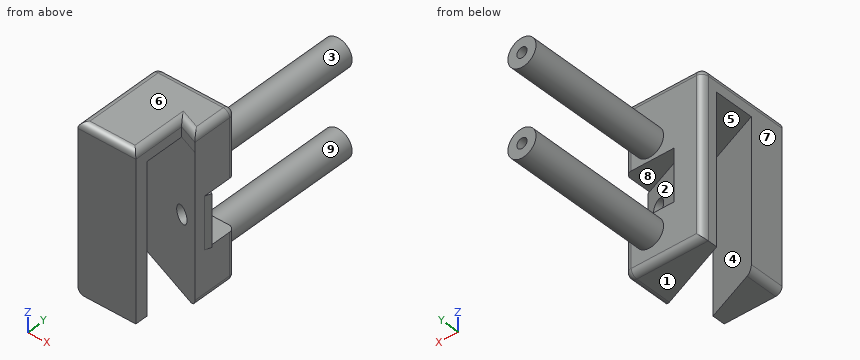
```python
from build123d import *

# Parameters (mm, degrees)
BOSS_EXTRUDE1_DEPTH  = 58.42
SKETCH2_W            = 22.86
SKETCH2_H            = 29.69248518
BOSS_EXTRUDE2_DEPTH  = 6.35
BOSS_EXTRUDE3_DEPTH  = 58.42
CUT_EXTRUDE1_DEPTH   = 58.42
BOSS_EXTRUDE5_DEPTH  = 19.05
BOSS_EXTRUDE6_DEPTH  = 19.05
SKETCH8_R            = 3.3
CUT_EXTRUDE2_DEPTH   = 4.085289
SKETCH9_R            = 5.55625
BOSS_EXTRUDE7_DEPTH  = 64.262
SKETCH11_R           = 1.999996
CUT_EXTRUDE3_DEPTH   = 6.99999997
BOSS_EXTRUDE8_DEPTH  = 6.35
BOSS_EXTRUDE9_DEPTH  = 6.35
FILLET3_R            = 2.54
BOSS_EXTRUDE10_START = 2.54
SKETCH15_W           = 20.926247949
SKETCH15_H           = 20.32
SKETCH15_R           = 3.3
BOSS_EXTRUDE10_DEPTH = 2.54


with BuildPart() as part:
    # Sketch1 → Boss-Extrude1 (new body)
    with BuildSketch(Plane.XY):
        Polygon((0, 0), (22.86, 0), (22.86, 5.08), (0, 13.97), align=None)
    extrude(amount=BOSS_EXTRUDE1_DEPTH)

    # Sketch2 → Boss-Extrude2 (add)
    with BuildSketch(Plane.XY.offset(58.42)):
        with Locations((11.43, 14.84624259)):
            Rectangle(SKETCH2_W, SKETCH2_H)
    extrude(amount=BOSS_EXTRUDE2_DEPTH)

    # Sketch3 → Boss-Extrude3 (add)
    with BuildSketch(Plane(origin=(0, 0, 58.42), x_dir=(-1, 0, 0), z_dir=(0, 0, -1))):
        Polygon((-22.86, 29.69248518), (0, 29.69248518), (-30.774794254, 17.724509637), (-30.774794254, 29.69248518), align=None)
    extrude(amount=BOSS_EXTRUDE3_DEPTH)

    # Sketch5 → Cut-Extrude1 (cut)
    with BuildSketch(Plane(origin=(0, 0, 0), x_dir=(-1, 0, 0), z_dir=(0, 0, -1))):
        Polygon((-30.774794254, 22.107844851), (-11.271433408, 29.69248518), (-30.774794254, 29.69248518), align=None)
    extrude(amount=-CUT_EXTRUDE1_DEPTH, mode=Mode.SUBTRACT)

    # Sketch7 → Boss-Extrude6 (add)
    with BuildSketch(Plane.XY.offset(58.42)):
        Polygon((30.774794254, 22.107844851), (30.774794254, 29.69248518), (11.271433408, 29.69248518), align=None)
    extrude(amount=-BOSS_EXTRUDE6_DEPTH)

    # Sketch8 → Cut-Extrude2 (cut)
    with BuildSketch(Plane(origin=(11.510866943, 29.599372139, 0), x_dir=(0.9320046715412958, -0.36244626115494866, 0), z_dir=(0.36244626115494866, 0.9320046715412958, 0))):
        with Locations(Location((13.92329977, -29.21, 0), (0, 0, 180))):
            Circle(SKETCH8_R)
    extrude(amount=-CUT_EXTRUDE2_DEPTH, mode=Mode.SUBTRACT)



with BuildPart() as body_2:
    # Sketch6 → Boss-Extrude5 (new body)
    with BuildSketch(Plane(origin=(0, 0, 0), x_dir=(-1, 0, 0), z_dir=(0, 0, -1))):
        Polygon((-30.774794254, 29.69248518), (-30.774794254, 22.107844851), (-11.271433408, 29.69248518), align=None)
    extrude(amount=-BOSS_EXTRUDE5_DEPTH)


with BuildPart() as part_1:
    add(part.part)

    add(body_2.part)  # Boss-Extrude7 merges body 2
    # Sketch9 → Boss-Extrude7 (add)
    with BuildSketch(Plane(origin=(0, 29.69248518, 0), x_dir=(1, 0, 0), z_dir=(0, 1, 0))):
        with Locations(Location((21.023113831, -12.065, 0), (0, 0, 270))):
            Circle(SKETCH9_R)
        with Locations(Location((21.023113831, -46.355, 0), (0, 0, 270))):
            Circle(SKETCH9_R)
    extrude(amount=BOSS_EXTRUDE7_DEPTH)

    # Sketch11 → Cut-Extrude3 (cut)
    with BuildSketch(Plane(origin=(0, 93.95448518, 0), x_dir=(1, 0, 0), z_dir=(0, 1, 0))):
        with Locations(Location((21.023113831, -12.065, 0), (0, 0, 270))):
            Circle(SKETCH11_R)
        with Locations(Location((21.023113831, -46.355, 0), (0, 0, 270))):
            Circle(SKETCH11_R)
    extrude(amount=-CUT_EXTRUDE3_DEPTH, mode=Mode.SUBTRACT)

    # Sketch12 → Boss-Extrude8 (add)
    with BuildSketch(Plane.XY.offset(58.42)):
        Polygon((22.86, 29.69248518), (30.774794254, 29.69248518), (30.774794254, 17.724509637), (22.86, 20.80248518), align=None)
    extrude(amount=BOSS_EXTRUDE8_DEPTH)

    # Sketch14 → Boss-Extrude9 (add)
    with BuildSketch(Plane(origin=(0, 29.69248518, 0), x_dir=(1, 0, 0), z_dir=(0, 1, 0))):
        Polygon((0, 0), (0, -64.77), (30.774794254, -64.77), (30.774794254, -39.37), (11.271433408, -39.37), (11.271433408, -19.05), (30.774794254, -19.05), (30.774794254, 0), align=None)
    extrude(amount=BOSS_EXTRUDE9_DEPTH)

    # Fillet3
    fillet3_edges = [part_1.edges().sort_by_distance(p)[0] for p in [
        (0, 18.02124259, 64.77),
        (15.387397127, 36.04248518, 64.77),
        (30.774794254, 26.883497409, 0),
        (30.774794254, 26.883497409, 64.77),
        (26.817397127, 19.263497409, 64.77),
        (22.86, 10.40124259, 64.77),
        (11.43, 0, 64.77),
        (0, 6.985, 0),
        (15.387397127, 36.04248518, 0),
        (0, 36.04248518, 32.385),
        (30.774794254, 36.04248518, 52.07),
        (30.774794254, 36.04248518, 9.525),
    ]]
    fillet(fillet3_edges, radius=FILLET3_R)

    # Sketch15 → Boss-Extrude10 (add)
    with BuildSketch(Plane(origin=(11.510866943, 29.599372139, 0), x_dir=(0.9320046715412958, -0.3624462611549486, 0), z_dir=(0.3624462611549486, 0.9320046715412958, 0)).offset(BOSS_EXTRUDE10_START)):
        with Locations((10.206222328, -29.21)):
            Rectangle(SKETCH15_W, SKETCH15_H)
        with Locations(Location((13.92329977, -29.21, 0), (0, 0, 180))):
            Circle(SKETCH15_R, mode=Mode.SUBTRACT)
    extrude(amount=-BOSS_EXTRUDE10_DEPTH)


solid = part_1.part
```
The model under review builds one solid part; all positions refer to its coordinate system, in mm. Face numbers are marked on the shaded views. A direction names the side the tool comes from. Round coordinates to 2 decimals unless told otherwise and drop trailing zeros. Loops run counter-clockwise (first coordinate to the right, second up) from the corner with the lowest first, then second, coordinate; pieces in that order, holes last.
1) Wall thickness on line 1 along Z through (x, y) = (21.5, 84); line 2 along Y through (x, z) = (14, 62); line 3 along Z through (x, y) = (25.5, 45.5): over which ranges is each line inside the solid? List them lowest first.
Values follow:
line 1: z = 6.53 to 17.6, 40.82 to 51.89
line 2: y = 0 to 36.04
line 3: z = 8.77 to 15.36, 43.06 to 49.65
2) The part is to be moulded in two halves that separate along Z. For the marked faces 6, 7, 8 and 9, say which applies: pulls with the +Z half, pulls with the -Z half, needs draft (parallel to the pull), parting line crosses it, or undercut.
Values follow:
face 6: pulls with the +Z half
face 7: needs draft
face 8: undercut
face 9: undercut
3) Consider section B-B on y = 15. State the section outline as (x, z) points, then the cut area to 3 significant figures.
Values follow:
outline: (0, 58.42) - (22.86, 58.42) - (22.86, 62.23) arc R2.54 ccw to (20.32, 64.77) - (2.54, 64.77) arc R2.54 ccw to (0, 62.23) - close
area: 142 mm2
4) Clearance check with flat-ended pins moving along their axes: P1, Ø1, axis at y = 15, z = 26.5, coming from the -X side; P2, Ø3, axis at x = 6.5, z = 36.5, coming from the +Y side; P3, Ø3.5, axis at x = 21.02, z = 46.36, coming from the +Y side; P4, Ø1, axis at x = 31, y = 24, coming from the +Z side. State where each tip first meets the part, or that it passes through.
Values follow:
P1: passes through
P2: stops at y = 36.04
P3: stops at y = 86.95
P4: stops at z = 63.38
5) Consider section A-A on z = 22. State the section outline as (x, y) points.
Values follow:
outline: (0, 0) - (22.86, 0) - (22.86, 5.08) - (0, 13.97) - close; (0, 29.69) - (30.77, 17.72) - (30.77, 22.11) - (31.7, 24.48) - (12.19, 32.06) - (11.27, 29.69) - (11.27, 36.04) - (2.54, 36.04) arc R2.54 ccw to (0, 33.5) - close
6) Consider section D-D on z = 57. State the section outline as (x, y) points.
Values follow:
outline: (0, 0) - (22.86, 0) - (22.86, 5.08) - (0, 13.97) - close; (0, 29.69) - (30.77, 17.72) - (30.77, 33.5) arc R2.54 ccw to (28.23, 36.04) - (2.54, 36.04) arc R2.54 ccw to (0, 33.5) - close
7) Tool access review of the marked faces 1, 2, 3, 4 and 5: name each direction out of +Z, -Z, +X, -X, +Y, -Y from which nothing blocks a thin tool from reaching the whole face with its end or side.
Values follow:
face 1: -Z, +X, -X, +Y, -Y
face 2: +X, +Y
face 3: +Y
face 4: -Z, +X
face 5: -Z
8) Consider section C-C on x = 8. State the section outline as (y, z) points, then the cut area to 3 significant figures.
Values follow:
outline: (0, 0) - (10.86, 0) - (10.86, 58.42) - (26.58, 58.42) - (26.58, 0) - (33.5, 0) arc R2.54 ccw to (36.04, 2.54) - (36.04, 62.23) arc R2.54 ccw to (33.5, 64.77) - (2.54, 64.77) arc R2.54 ccw to (0, 62.23) - close
area: 1,410 mm2
